Autodesk Inventor part; units mm, degrees
ref_plane "YZ Plane" through (0, 0, 0) normal (1, 0, 0) x (0, 1, 0)
ref_plane "XZ Plane" through (0, 0, 0) normal (0, 1, 0) x (-1, 0, 0)
ref_plane "XY Plane" through (0, 0, 0) normal (0, 0, 1) x (1, 0, 0)
sketch "Sketch1" plane through (0, 0, 0) normal (0, 0, 1) x (1, 0, 0)
  line L0 (0, 31.75) -> (4.1656, 31.75)
  line L1 (4.1656, 31.75) -> (4.1656, 0)
  line L2 (4.1656, 0) -> (0, 0)
  line L3 (0, 0) -> (0, 31.75)
  line L4 (4.1656, 0) -> (14.8844, 0)
  line L5 (14.8844, 0) -> (14.8844, 4.1656)
  line L6 (14.8844, 4.1656) -> (4.1656, 4.1656)
  line L7 (4.1656, 4.1656) -> (4.1656, 0)
  line L8 (14.8844, 4.1656) -> (19.05, 4.1656)
  line L9 (19.05, 4.1656) -> (19.05, -17.161)
  line L10 (19.05, -17.161) -> (14.8844, -17.161)
  line L11 (14.8844, -17.161) -> (14.8844, 4.1656)
  arc A0 (14.8844, -17.161) -> (33.9344, -26.2503) centre (26.5778, -17.161) ccw
  arc A1 (19.05, -17.161) -> (31.3137, -23.0124) centre (26.5778, -17.161) ccw
  line L12 (33.9344, -26.2503) -> (31.3137, -23.0124)
  line L13 (16.255, -28.8544) -> (45.3124, -28.8544)
  dimension "d0" = 31.75
  dimension "d1" = 19.05
  dimension "d2" = 4.1656
  dimension "d5" = 33.02
  dimension "d6" = 19.05
  dimension "d7" = 5.842
extrude "Extrusion1" add sketch "Sketch1" along normal blind 381
sketch "Sketch2" plane through (0, 0, 0) normal (0, 0, -1) x (-1, 0, 0)
  line L0 (0, 31.75) -> (0, 0)
  line L1 (-4.1656, 31.75) -> (0, 31.75)
  line L2 (-4.1656, 4.1656) -> (-4.1656, 31.75)
  arc A0 (-33.9344, -26.2503) -> (-14.8844, -17.161) centre (-26.5778, -17.161) ccw
  line L3 (-31.75, 38.5572) -> (-6.8072, 38.5572)
  line L4 (-6.8072, 38.5572) -> (-6.8072, 34.3916)
  line L5 (-6.8072, 34.3916) -> (-31.75, 34.3916)
  line L6 (-31.75, 34.3916) -> (-31.75, 38.5572)
  arc A1 (0, 31.75) -> (-6.8072, 38.5572) centre (-6.8072, 31.75) ccw
  arc A2 (-4.1656, 31.75) -> (-6.8072, 34.3916) centre (-6.8072, 31.75) ccw
  line L7 (-19.05, -28.8544) -> (-58.4387, -28.8544)
  dimension "d12" = 67.4116
  dimension "d13" = 31.75
extrude "Extrusion2" add sketch "Sketch2" against normal blind 314.325
fillet "Fillet1" radius 9.525 1 edges at (31.75, 36.4744, 314.325)
ref_plane "Work Plane1" through (177.8, 0, 381) normal (-1, 0, 0) x (0, 0, 1)
sketch "Sketch4" plane through (4.1656, 4.1656, 381) normal (1, 0, 0) x (0, 0, -1)
  line L0 (66.675, 27.5844) -> (0, 27.5844)
  line L1 (0, 27.5844) -> (0, 0)
  point P0 (381, -4.1656)
  point P1 (40, 11.7094)
  dimension "d24" = 15.875
  dimension "d25" = 40
hole "Hole1" at (4.1656, 15.875, 341) direction (-1, 0, 0) diameter 6.35 end through all
mirror "Mirror2" about plane through (177.8, 0, 381) normal (-1, 0, 0) of "Extrusion1", "Extrusion2", "Fillet1", "Hole1"
sketch "Sketch3" plane through (19.05, -17.161, 0) normal (1, 0, 0) x (0, 0, -1)
  line L0 (0, 0) -> (0, 21.3266)
  line L1 (0, 21.3266) -> (-381, 21.3266)
  line L2 (0, -4.0734) -> (5.08, -4.0734)
  line L3 (5.08, -4.0734) -> (5.08, 21.3266)
  line L4 (5.08, 21.3266) -> (0, 21.3266)
  line L5 (0, 21.3266) -> (0, -4.0734)
  line L6 (5.08, 21.3266) -> (25.4, 21.3266)
  line L7 (25.4, 21.3266) -> (25.4, 16.2466)
  line L8 (25.4, 16.2466) -> (5.08, 16.2466)
  line L9 (5.08, 16.2466) -> (5.08, 21.3266)
  point P0 (0, 17.161)
  dimension "d18" = 5.08
  dimension "d19" = 25.4
  dimension "d20" = 25.4
extrude "crosspiece" add sketch "Sketch3" along normal up to surface (317.5 mm away)
properties part number "battery rails"
Can you work these out from the model? Positions are in its coordinate system, mm. A direction names the side the tool comes from. Coordinates: 2 decimals unless noted, no trailing zeros. Write each loop counter-clockwise with the first axis right and the second up, starting at its lowest first coordinate (ties: lowest second). Pieces come first, ordered by that corner, then holes. Notation, with made-up numbers: M 60,87.5 L 95,87.5 A22 ccw 95,117.5 Z; hole C 15,6.5 d10. An arc over 180 degrees is marked long. Answer as CSV lines item,"result".
Item 1: I'm going to push flat-ended pins straight in: P1, Ø5.5, axis at x = 13, y = 35.5, coming from the +Z side (3 decimals); P2, Ø5.5, axis at y = 15.875, z = 341, coming from the -X side; P3, Ø6, axis at x = 228.5, z = -18.5, coming from the -Y side; P4, Ø1.5, axis at x = 151.5, y = -18.5, coming from the -Z side. Where does each tip first touch, or does it pass through?
Geometry results:
P1,"stops at z = 314.325"
P2,"passes through"
P3,"stops at y = -0.91"
P4,"stops at z = -5.08"
Item 2: On a 3-axis mill with a long thin cutter (end or side, diameter ignored), from which of +Z, -Z, +X, -X, +Y, -Y can I reach the whole of each face in a straight line? I mean faces 1 (the cylindrical face through (28.886, 36.504, 311.609)), 2 (the cylindrical face through (23.444, -24.005, 187.833)), 3 (the flat face through (348, 0, 188)), 4 (the flat face through (4.166, 18, 188)), 5 (the flat face through (176, -0.914, -15)). Say none if no direction works.
Geometry results:
face 1,"+Z, +Y"
face 2,"+Z"
face 3,"+Z, -Z, +X, -Y"
face 4,"+Z, -Z"
face 5,"-Z, +X, -X, -Y"
Item 3: We'd pull the mould along Y, two halves only. Please class faces 6 (the flat face through (176, 4.166, -13)), 7 (the flat face through (336.55, 0, -7)), 8 (the cylindrical face through (21.709, -27.793, 187.833)), 9 (the flat face through (12, 4.166, 188)): +Y half, -Y half, draft (parallel to the pull), parting line (faces both ways), or undercut.
Geometry results:
face 6,"+Y half"
face 7,"draft"
face 8,"-Y half"
face 9,"undercut"
Item 4: Imagine slicing it at B-B on x = 161. List the corners of the cut face in (y, z) for me, plus the area to 3 significant figures.
Geometry results:
outline,"M -21.23,-5.08 L -0.91,-5.08 L -0.91,-25.4 L 4.17,-25.4 L 4.17,0 L -21.23,0 Z"
area,"232 mm2"
Item 5: Please list where these lines run through material, in increasing order: line 1 along X through (y, z) = (-9.5, 334); line 2 along Y through (x, z) = (354.5, 341); line 3 along X through (y, z) = (8, 277).
Geometry results:
line 1,"x = 14.88 to 19.05, 336.55 to 340.72"
line 2,"y = 0 to 12.7, 19.05 to 31.75"
line 3,"x = 0 to 4.17, 351.43 to 355.6"
Item 6: Imagine slicing it at A-A on z = 264. List the corners of the cut face in (x, y) for me.
Geometry results:
outline,"M 0,0 L 14.88,0 L 14.88,-17.16 A11.69 ccw 33.93,-26.25 L 31.31,-23.01 A7.53 cw 19.05,-17.16 L 19.05,4.17 L 4.17,4.17 L 4.17,31.75 A2.64 cw 6.81,34.39 L 31.75,34.39 L 31.75,38.56 L 6.81,38.56 A6.81 ccw 0,31.75 Z; M 321.67,-26.25 A11.69 ccw 340.72,-17.16 L 340.72,0 L 355.6,0 L 355.6,31.75 A6.81 ccw 348.79,38.56 L 323.85,38.56 L 323.85,34.39 L 348.79,34.39 A2.64 cw 351.43,31.75 L 351.43,4.17 L 336.55,4.17 L 336.55,-17.16 A7.53 cw 324.29,-23.01 Z"
